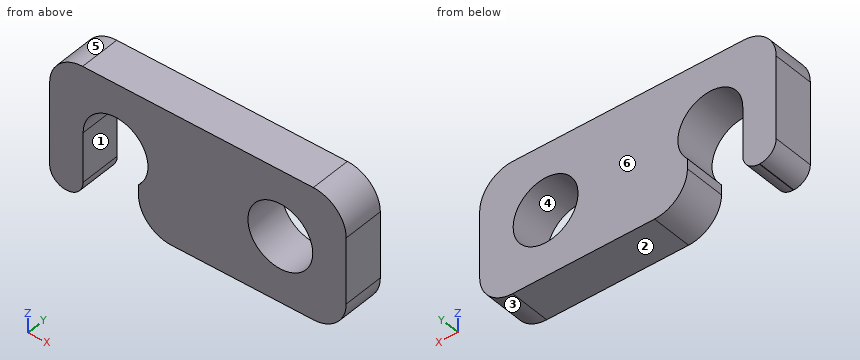
```python
from build123d import *

# Parameters (mm, degrees)
SKETCH1_W           = 22.86
SKETCH1_H           = 10.16
BOSS_EXTRUDE1_DEPTH = 3.175
SKETCH2_R           = 2.5
CUT_EXTRUDE1_DEPTH  = 4.175
CUT_EXTRUDE2_DEPTH  = 4.175
FILLET1_R           = 2.54
FILLET2_R           = 1.27


with BuildPart() as part:
    # Sketch1 → Boss-Extrude1 (new body)
    with BuildSketch(Plane(origin=(0, 0, 0), x_dir=(1, 0, 0), z_dir=(0, 1, 0))):
        Rectangle(SKETCH1_W, SKETCH1_H)
    extrude(amount=BOSS_EXTRUDE1_DEPTH)

    # Sketch2 → Cut-Extrude1 (cut, through all)
    with BuildSketch(Plane(origin=(0, 3.175, 0), x_dir=(1, 0, 0), z_dir=(0, 1, 0))):
        with Locations((-6.35, 0)):
            Circle(SKETCH2_R)
        with Locations((6.35, 0)):
            Circle(SKETCH2_R)
    extrude(amount=-CUT_EXTRUDE1_DEPTH, mode=Mode.SUBTRACT)

    # Sketch3 → Cut-Extrude2 (cut, through all)
    with BuildSketch(Plane(origin=(0, 3.175, 0), x_dir=(1, 0, 0), z_dir=(0, 1, 0))):
        with BuildLine():
            Line((-8.85, 0), (-8.85, 5.08))
            Line((-8.85, 5.08), (-4.584545949, 5.08))
            Line((-4.584545949, 5.08), (-4.584545949, 1.770076833))
            ThreePointArc((-4.584545949, 1.770076833), (-7.308218366, 2.30907288), (-8.85, 0))
        make_face()
    extrude(amount=-CUT_EXTRUDE2_DEPTH, mode=Mode.SUBTRACT)

    # Fillet1
    fillet1_edges = [part.edges().sort_by_distance(p)[0] for p in [
        (-4.584545949, 1.5875, -5.08),
        (11.43, 1.5875, 5.08),
        (-11.43, 1.5875, 5.08),
        (11.43, 1.5875, -5.08),
    ]]
    fillet(fillet1_edges, radius=FILLET1_R)

    # Fillet2
    fillet2_edges = [part.edges().sort_by_distance(p)[0] for p in [
        (-8.85, 1.5875, -5.08),
        (-11.43, 1.5875, -5.08),
    ]]
    fillet(fillet2_edges, radius=FILLET2_R)


solid = part.part
```
For this review, take the finished solid that the model builds, in its own axes (mm). Face numbers are marked on the shaded views. A direction names the side the tool comes from. Round coordinates to 2 decimals unless told otherwise and drop trailing zeros. Write each loop counter-clockwise with the first axis right and the second up, starting at its lowest first coordinate (ties: lowest second). Pieces come first, ordered by that corner, then holes.
1) Take a section at A-A on x = 6.35. Give the boundary of the cut face in (y, z) (3 decimals), then the cut area to 3 significant figures.
Answer below:
outline: (0, -5.08) - (3.175, -5.08) - (3.175, -2.5) - (0, -2.5) - close; (0, 2.5) - (3.175, 2.5) - (3.175, 5.08) - (0, 5.08) - close
area: 16.4 mm2
2) Take a section at D-D on z = 2.25. Give the boundary of the cut face in (x, y) (3 decimals), then the cut area to 3 significant figures.
Answer below:
outline: (-11.43, 0) - (-7.44, 0) - (-7.44, 3.175) - (-11.43, 3.175) - close; (-5.26, 0) - (5.26, 0) - (5.26, 3.175) - (-5.26, 3.175) - close; (7.44, 0) - (11.43, 0) - (11.43, 3.175) - (7.44, 3.175) - close
area: 58.7 mm2
3) Take a section at B-B on y = 1.65. Give the boundary of the cut face in (x, z), then the cut area to 3 significant figures.
Answer below:
outline: (-11.43, -3.81) arc R1.27 ccw to (-10.16, -5.08) - (-10.12, -5.08) arc R1.27 ccw to (-8.85, -3.81) - (-8.85, 0) arc R2.5 cw (long way) to (-4.58, -1.77) - (-4.58, -2.54) arc R2.54 ccw to (-2.04, -5.08) - (8.89, -5.08) arc R2.54 ccw to (11.43, -2.54) - (11.43, 2.54) arc R2.54 ccw to (8.89, 5.08) - (-8.89, 5.08) arc R2.54 ccw to (-11.43, 2.54) - close; hole circle Ø5 at (6.35, 0)
area: 174 mm2
4) Take a section at C-C on z = 1. Give the boundary of the cut face in (x, y) (3 decimals).
Answer below:
outline: (-11.43, 0) - (-8.641, 0) - (-8.641, 3.175) - (-11.43, 3.175) - close; (-4.059, 0) - (4.059, 0) - (4.059, 3.175) - (-4.059, 3.175) - close; (8.641, 0) - (11.43, 0) - (11.43, 3.175) - (8.641, 3.175) - close
5) For line 1 along Z through (x, y) = (6.35, 2); line 2 along X through (y, z) = (2.35, -0.5); line 3 along X through (y, z) = (2.65, -1.75), list the stretches that pass through material, from the lowest coordinate up.
Answer below:
line 1: z = -5.08 to -2.5, 2.5 to 5.08
line 2: x = -11.43 to -8.85, -3.9 to 3.9, 8.8 to 11.43
line 3: x = -11.43 to -8.85, -4.56 to 4.56, 8.14 to 11.43
6) Machinability: for the marked faces 1 and 2, which of the approach directions +Z, -Z, +X, -X, +Y, -Y give a long, thin tool a straight path to every point of the face, cutting with its end or side? Answer none if there is none.
Answer below:
face 1: -Z, +Y, -Y
face 2: -Z, +X, -X, +Y, -Y
7) Mouldability with a two-part tool opening along X and no side actions: class the marked faces 3, 4, 5 and 6 as +X half, -X half, draft (parallel to the pull), parting line (faces both ways), or undercut.
Answer below:
face 3: +X half
face 4: undercut
face 5: -X half
face 6: draft
